Verification items for the finished model (mm, model axes). Face numbers are marked on the shaded views. A direction names the side the tool comes from. Coordinates: 2 decimals unless noted, no trailing zeros. Order: outer loops, then holes, each group sorted by start corner. A loop starts at its lowest first (then second) coordinate and runs counter-clockwise, first axis right, second up. Notation, with made-up numbers: M 53.25,-6.5 L 88.25,-6.5 A19 ccw 88.25,19.5 Z; hole C -15,84 d2. An arc over 180 degrees is marked long. Answer as a JSON object with one key per item and string values. Group by question number.
(1) Material ranges on line 1 (Z direction, x = 1.25, y = -5); line 2 (Y direction, x = -1.5, z = -1.5), recorded low to high.
(2) Cross-section at A-A (z = -1). Enter the section's corners in (x, y).
(3) Cross-section at B-B (y = -4). Enter the section's corners in (x, z).
(4) Cross-section at D-D (y = -1). Enter the section's corners in (x, z), plus the area to 3 significant figures.
(5) Access from +Z, -Z, +X, -X, +Y, -Y to the whole of each face (thin tool, end or side, straight path). Record for the marked faces 1 and 2.
(6) Gauge pin test, flat ends, axial feed: pin 1 Ø5 at (x, y) = (1.5, -4.5) entering from -Z; pin 2 Ø1 at (x, y) = (0, -3.5) entering from -Z. Record the tip position at first contact, or that the pin passes through.
(7) Cross-section at C-C (x = 3.75). Enter the section's corners in (y, z), plus the area to 3 significant figures.
(8) Mould release check, pull along X, two halves, no side actions. Record for the marked faces 3, 4 and 5: released by +X, released by -X, zero draft, split by the parting line, or undercut.
from build123d import *

# Parameters (mm, degrees)
SKETCH1_W           = 10.7
SKETCH1_H           = 11
BOSS_EXTRUDE1_DEPTH = 5.9
SKETCH2_R           = 0.45
BOSS_EXTRUDE2_DEPTH = 3.4


with BuildPart() as part:
    # Sketch1 → Boss-Extrude1 (new body)
    with BuildSketch(Plane.XY):
        Rectangle(SKETCH1_W, SKETCH1_H)
    extrude(amount=BOSS_EXTRUDE1_DEPTH)

    # Sketch2 → Boss-Extrude2 (add)
    with BuildSketch(Plane(origin=(0, 0, 0), x_dir=(-1, 0, 0), z_dir=(0, 0, -1))):
        with Locations((-3.75, -4)):
            Circle(SKETCH2_R)
        with Locations((-1.25, -4)):
            Circle(SKETCH2_R)
        with Locations((1.25, -4)):
            Circle(SKETCH2_R)
        with Locations((3.75, -4)):
            Circle(SKETCH2_R)
    extrude(amount=BOSS_EXTRUDE2_DEPTH)


solid = part.part
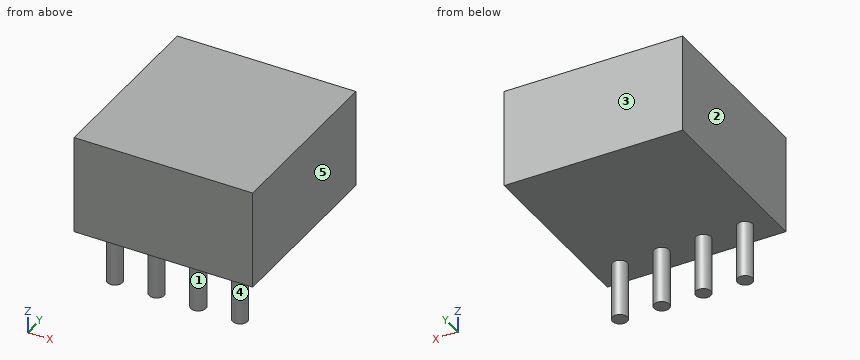
Taken from the geometry:
{
 "1": {"line 1": "z = 0 to 5.9", "line 2": "y = -4.37 to -3.63"},
 "2": {"outline": "C -3.75,-4 d0.9; C -1.25,-4 d0.9; C 1.25,-4 d0.9; C 3.75,-4 d0.9"},
 "3": {"outline": "M -5.35,0 L -4.2,0 L -4.2,-3.4 L -3.3,-3.4 L -3.3,0 L -1.7,0 L -1.7,-3.4 L -0.8,-3.4 L -0.8,0 L 0.8,0 L 0.8,-3.4 L 1.7,-3.4 L 1.7,0 L 3.3,0 L 3.3,-3.4 L 4.2,-3.4 L 4.2,0 L 5.35,0 L 5.35,5.9 L -5.35,5.9 Z"},
 "4": {"outline": "M -5.35,0 L 5.35,0 L 5.35,5.9 L -5.35,5.9 Z", "area": "63.1 mm²"},
 "5": {"face 1": "-Z", "face 2": "+Z, -Z, -X, +Y, -Y"},
 "6": {"pin 1": "stops at z = -3.4", "pin 2": "stops at z = 0"},
 "7": {"outline": "M -5.5,0 L -4.45,0 L -4.45,-3.4 L -3.55,-3.4 L -3.55,0 L 5.5,0 L 5.5,5.9 L -5.5,5.9 Z", "area": "68.0 mm²"},
 "8": {"face 3": "zero draft", "face 4": "undercut", "face 5": "released by +X"}
}
